from build123d import *

# Parameters (mm, degrees)
F0_W     = 57.15
F0_H     = 38.1
F1_DEPTH = 25.4
F2_W     = 15.875
F2_H     = 7.62
F3_DEPTH = 19.05
F4_R     = 12.7
F5_DEPTH = 25.401
F6_R     = 5.08
F7_R     = 5.08


with BuildPart() as f1:
    # F0 (on Top) → F1 (new body)
    with BuildSketch(Plane.XY):
        Rectangle(F0_W, F0_H)
    extrude(amount=F1_DEPTH)

    # F2 (on face) → F3 (cut)
    with BuildSketch(Plane.XY.offset(25.4)):
        with Locations((-7.9375, -15.24)):
            Rectangle(F2_W, F2_H)
        with Locations((7.9375, -15.24)):
            Rectangle(F2_W, F2_H)
        Polygon((-28.575, 19.05), (-28.575, -19.05), (-22.225, -19.05), (-22.225, 0), (-15.875, 0), (-15.875, 19.05), (-22.225, 19.05), align=None)
        Polygon((22.225, 19.05), (15.875, 19.05), (15.875, 0), (22.225, 0), (22.225, -19.05), (28.575, -19.05), (28.575, 19.05), align=None)
    extrude(amount=-F3_DEPTH, mode=Mode.SUBTRACT)

    # F4 (on face) → F5 (cut, through all)
    with BuildSketch(Plane.XY.offset(25.4)):
        with Locations((0, 19.05)):
            Circle(F4_R)
    extrude(amount=-F5_DEPTH, mode=Mode.SUBTRACT)

    # F6
    f6_edges = [f1.edges().sort_by_distance(p)[0] for p in [
        (-15.875, 0, 15.875),
        (15.875, 0, 15.875),
    ]]
    fillet(f6_edges, radius=F6_R)

    # F7
    f7_edges = [f1.edges().sort_by_distance(p)[0] for p in [
        (28.575, 19.05, 3.175),
        (-28.575, 19.05, 3.175),
    ]]
    fillet(f7_edges, radius=F7_R)


solid = f1.part
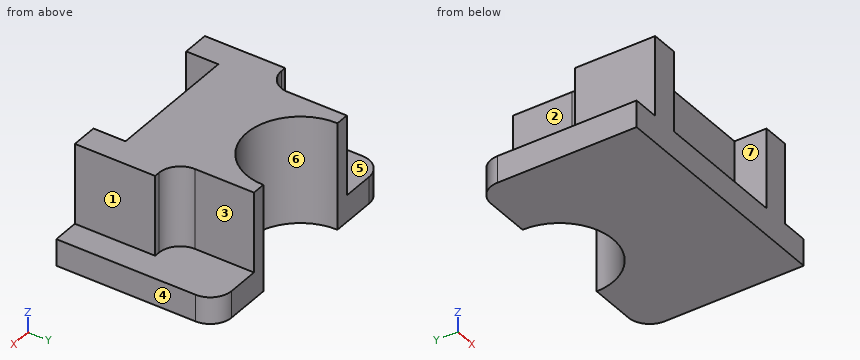
Model file for the job. Use its own axes, mm. Face numbers are marked on the shaded views. A direction names the side the tool comes from. Coordinates: 2 decimals unless noted, no trailing zeros. Write each loop counter-clockwise with the first axis right and the second up, starting at its lowest first coordinate (ties: lowest second). Pieces come first, ordered by that corner, then holes. Notation, with made-up numbers: (-9, -33.75) - (-5, -33.75) arc R28 ccw to (-5, -4.75) - close; hole circle Ø10 at (19.25, -6). An arc over 180 degrees is marked (long way). Write each question's results on one line, items separated by ' | '. Start each with the question number.
1) 3-axis set-ups, long thin cutter, end or side, ignore diameter. For the marked faces 1, 2 and 3: which of +Z, -Z, +X, -X, +Y, -Y reach the whole face in a straight line?
2) Flat gauge pins, fed straight in: P1, Ø9.5, axis at y = -14, z = 11.5, coming from the +X side (3 decimals); P2, Ø8.5, axis at y = -16, z = 11, coming from the -X side (3 decimals); P3, Ø1.4, axis at x = -21.5, z = 16.5, coming from the +Y side. Where does each tip first touch, or does it go through?
3) Probe line 1 along X through (y, z) = (-13.5, 19.75) (3 decimals); line 2 along Z through (x, y) = (-25.5, -8.5); line 3 along X through (y, z) = (5, 15.5). List the from-to ranges inside material, lowest first. Write a range as from..to.
4) Mould opens along X. For the marked faces 4, 5, 6 and 7 say: pulls with the +X half, pulls with the -X half, needs draft (parallel to the pull), parting line crosses it, or undercut.
5) Cut at A-A (z = 3). Write the cut outline in (x, y) (3 decimals), then the cut area to 3 significant figures.
6) Cut at D-D (z = 10.75). Write the cut outline in (x, y) (3 decimals), then the cut area to 3 significant figures.
7) Cut at B-B (x = 0). Write the cut outline in (y, z).
Returned:
1) face 1: +Z, +X, +Y, -Y | face 2: +Z, -X, +Y | face 3: +Z, +X, +Y
2) P1: x = 22.225 | P2: x = -22.225 | P3: y = 0
3) line 1: -22.225..-15.875, 15.875..22.225 | line 2: 0..6.35 | line 3: -15.88..15.88
4) face 4: pulls with the +X half | face 5: needs draft | face 6: undercut | face 7: undercut
5) outline: (-28.575, -19.05) - (28.575, -19.05) - (28.575, 13.97) arc R5.08 ccw to (23.495, 19.05) - (12.7, 19.05) arc R12.7 cw to (-12.7, 19.05) - (-23.495, 19.05) arc R5.08 ccw to (-28.575, 13.97) - close | area: 1,910 mm^2
6) outline: (-22.225, -19.05) - (-15.875, -19.05) - (-15.875, -11.43) - (15.875, -11.43) - (15.875, -19.05) - (22.225, -19.05) - (22.225, 0) - (20.955, 0) arc R5.08 cw to (15.875, 5.08) - (15.875, 19.05) - (12.7, 19.05) arc R12.7 cw to (-12.7, 19.05) - (-15.875, 19.05) - (-15.875, 5.08) arc R5.08 cw to (-20.955, 0) - (-22.225, 0) - close | area: 967 mm^2
7) outline: (-19.05, 0) - (6.35, 0) - (6.35, 25.4) - (-11.43, 25.4) - (-11.43, 6.35) - (-19.05, 6.35) - close
